from build123d import *

# Parameters (mm, degrees)
SKETCH004_R     = 1.25
POCKET_DEPTH    = 10.001
PAD_DEPTH       = 2.5
POCKET005_DEPTH = 12


with BuildPart() as part:
    # Sketch → AdditiveLoft section 0
    with BuildSketch(Plane.XY):
        Polygon((0, 5.773503), (-5, 2.886751), (-5, -2.886751), (0, -5.773503), (5, -2.886751), (5, 2.886751), align=None)
    # Sketch001 (on DatumPlane) → AdditiveLoft section 1
    with BuildSketch(Plane.XY.offset(10)):
        Polygon((-5.773503, 10), (-11.547005, 0), (-5.773503, -10), (5.773503, -10), (11.547005, 0), (5.773503, 10), align=None)
    loft()

    # Sketch004 → Pocket (cut, through all)
    with BuildSketch(Plane.XY):
        Circle(SKETCH004_R)
    extrude(amount=POCKET_DEPTH, mode=Mode.SUBTRACT)

    # Sketch020 (on DatumPlane) → Pad (join, symmetric)
    with BuildSketch(Plane(origin=(0, 0, 10), x_dir=(0, 1, 0), z_dir=(1, 0, 0))):
        with BuildLine():
            ThreePointArc((-3.3, 4.5), (-3.55, 4.25), (-3.3, 4))
            Line((-3.3, 4), (-3.3, 1))
            Line((-3.3, 1), (-4.3, 0))
            Line((-4.3, 0), (-1.5, 0))
            Line((-1.5, 0), (-2.5, 1))
            Line((-2.5, 4.5), (-2.5, 1))
            Line((-3.3, 4.5), (-2.5, 4.5))
        make_face()
        with BuildLine():
            Line((4.3, 0), (1.5, 0))
            Line((2.5, 1), (1.5, 0))
            Line((2.5, 4.5), (2.5, 1))
            Line((3.3, 4.5), (2.5, 4.5))
            ThreePointArc((3.3, 4), (3.55, 4.25), (3.3, 4.5))
            Line((3.3, 1), (3.3, 4))
            Line((4.3, 0), (3.3, 1))
        make_face()
    extrude(amount=PAD_DEPTH, both=True)

    # Sketch017 (on DatumPlane) → Pocket005 (cut)
    with BuildSketch(Plane.XY.offset(14.5)):
        Polygon((1.212436, 2.1), (-1.212436, 2.1), (-2.424871, 0), (-1.212436, -2.1), (1.212436, -2.1), (2.424871, 0), align=None)
    extrude(amount=-POCKET005_DEPTH, mode=Mode.SUBTRACT)


solid = part.part
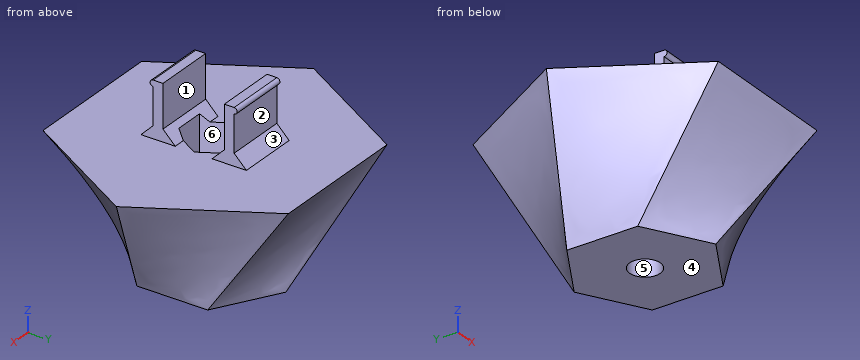
Verification items for the finished model (mm, model axes). Face numbers are marked on the shaded views. A direction names the side the tool comes from. Give positions to 0.01 mm unless a question says otherwise; leave off trailing zeros.
(1) Material ranges on line 1 (X direction, y = 0, z = 1.75); line 2 (X direction, y = 0, z = 2); line 3 (Y direction, x = 0, z = 0.8), recorded low to high.
(2) Mould release check, pull along Z, two halves, no side actions. Record for the marked faces 1, 2, 3 and 4: +Z half, -Z half, draft (parallel to the pull), parting line (faces both ways), or undercut.
(3) Gauge pin test, flat ends, axial feed: pin 1 (1.5 mm diameter, centred on x = 8.5, y = -0.5, fed in from +Z); pin 2 (1 mm diameter, centred on x = -1, z = 12.5, fed in from -Y); pin 3 (0.8 mm diameter, centred on y = 3, z = 13, fed in from +X). Record the tip position at first contact, or that the pin passes through.
(4) Access from +Z, -Z, +X, -X, +Y, -Y to the whole of each face (thin tool, end or side, straight path). Record for the marked faces 5 and 6.
Worked out:
1. line 1: x = -5.78 to -1.25, 1.25 to 5.78
1. line 2: x = -5.91 to -1.25, 1.25 to 5.91
1. line 3: y = -5.89 to -1.25, 1.25 to 5.89
2. face 1: draft
2. face 2: undercut
2. face 3: undercut
2. face 4: -Z half
3. pin 1: stops at z = 10
3. pin 2: stops at y = -3.3
3. pin 3: stops at x = 2.5
4. face 5: +Z, -Z
4. face 6: +Z
